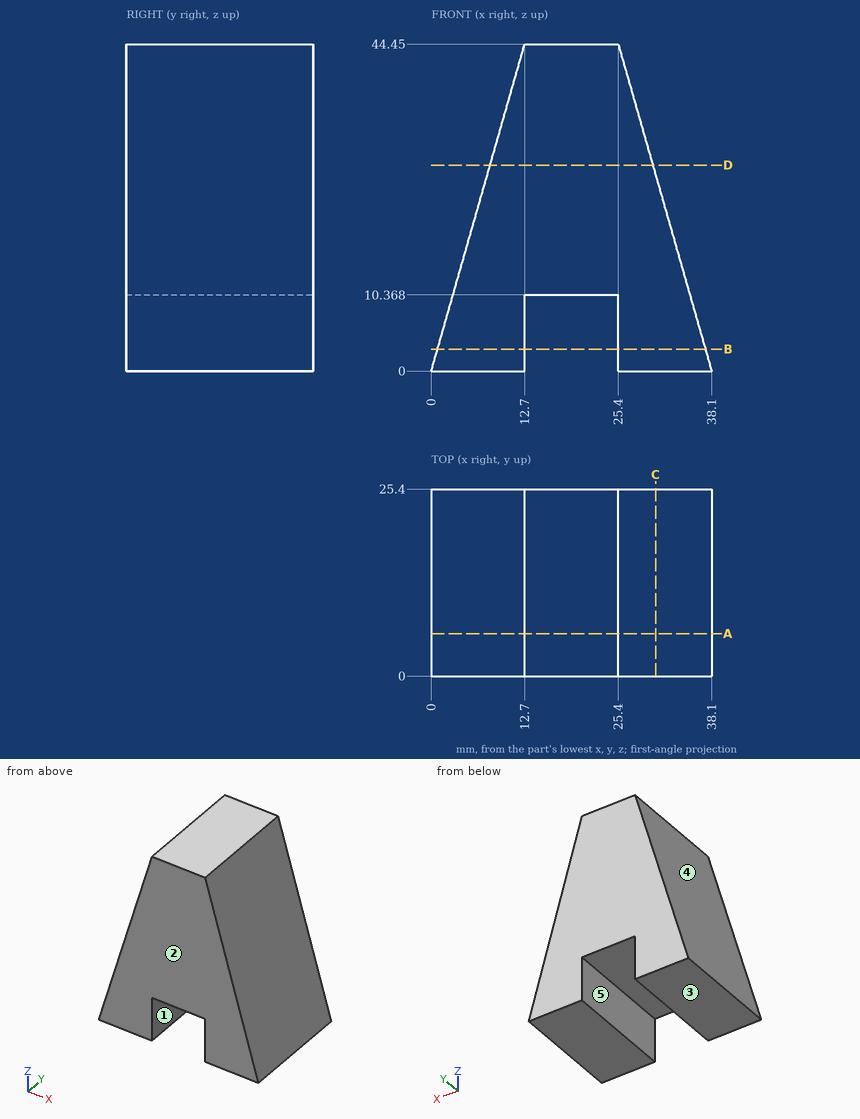
For this review, use the dimensioned drawing (mm, ordinates from the lowest corner) and the shaded views. A direction names the side the tool comes from. Give positions to 0.01 mm unless a question says otherwise; leave off trailing zeros. Loops run counter-clockwise (first coordinate to the right, second up) from the corner with the lowest first, then second, coordinate; pieces in that order, holes last.
Item 1: For line 1 along Z through (x, y) = (18.5, 6.5); line 2 along X through (y, z) = (10, 4.5) (1 decimal); line 3 along X through (y, z) = (23, 9), list the stretches that pass through material, from the lowest coordinate up.
Item 2: Take a section at B-B, the plane z = 3. State the section outline as (x, y) points, and give its area (3 significant figures).
Item 3: Insertion check: pin 1 (5 mm diameter, centred on y = 18, z = 34.5, fed in from +X); pin 2 (1 mm diameter, centred on y = 14, z = 31, fed in from -X); pin 3 (11.5 mm diameter, centred on y = 9.5, z = 7, fed in from +X). Each pin has a flat end and moves straight along its axis. Give the tip position at first contact, or say it passes through.
Item 4: Draft analysis for pull direction X (two halves, no side actions). For the marked faces 3, 4 and 5, state which applies: +X half, -X half, draft (parallel to the pull), parting line (faces both ways), or undercut.
Item 5: Tool access review of the marked faces 1 and 2: name each direction out of +Z, -Z, +X, -X, +Y, -Y from which nothing blocks a thin tool from reaching the whole face with its end or side.
Item 6: Take a section at D-D, the plane z = 28. State the section outline as (x, y) points, and give its area (3 significant figures).
Item 7: Take a section at A-A, the plane y = 5.75. State the section outline as (x, z) points, and give its area (3 significant figures).
Item 8: Take a section at C-C, the plane x = 30.5. State the section outline as (y, z) points.
Calculated:
1. line 1: z = 10.37 to 44.45
1. line 2: x = 1.3 to 12.7, 25.4 to 36.8
1. line 3: x = 2.57 to 12.7, 25.4 to 35.53
2. outline: (0.86, 0) - (12.7, 0) - (12.7, 25.4) - (0.86, 25.4) - close; (25.4, 0) - (37.24, 0) - (37.24, 25.4) - (25.4, 25.4) - close
2. area: 602 mm2
3. pin 1: stops at x = 28.96
3. pin 2: stops at x = 8.71
3. pin 3: stops at x = 37.74
4. face 3: draft
4. face 4: -X half
4. face 5: undercut
5. face 1: -Z, +Y, -Y
5. face 2: +Z, -Z, +X, -X, -Y
6. outline: (8, 0) - (30.1, 0) - (30.1, 25.4) - (8, 25.4) - close
6. area: 561 mm2
7. outline: (0, 0) - (12.7, 0) - (12.7, 10.37) - (25.4, 10.37) - (25.4, 0) - (38.1, 0) - (25.4, 44.45) - (12.7, 44.45) - close
7. area: 997 mm2
8. outline: (0, 0) - (25.4, 0) - (25.4, 26.6) - (0, 26.6) - close
